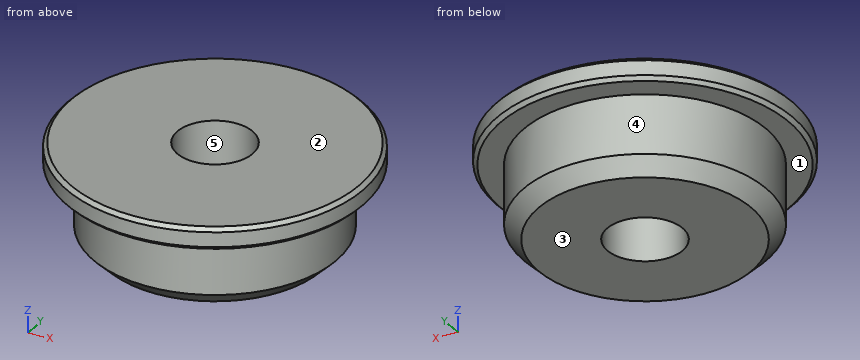
Autodesk Inventor part; units mm, degrees
ref_plane "YZ Plane" through (0, 0, 0) normal (1, 0, 0) x (0, 1, 0)
ref_plane "XZ Plane" through (0, 0, 0) normal (0, 1, 0) x (-1, 0, 0)
ref_plane "XY Plane" through (0, 0, 0) normal (0, 0, 1) x (1, 0, 0)
sketch "スケッチ1" plane through (0, 0, 0) normal (0, 0, 1) x (1, 0, 0)
  circle A0 centre (0, 0) radius 16.4
  dimension "d0" = 32.8
extrude "押し出し1" add sketch "スケッチ1" along normal blind 10
sketch "スケッチ2" plane through (0, 0, 10) normal (0, 0, 1) x (1, 0, 0)
  circle A0 centre (0, 0) radius 16.4
  circle A1 centre (0, 0) radius 20
  dimension "d3" = 40
extrude "押し出し2" add sketch "スケッチ2" along normal blind 3 contours A0 | A1
chamfer "面取り1" distance 2 angle 45 1 edges at (-16.4, 0, 0)
chamfer "面取り2" distance 0.5 angle 45 2 edges at (-20, 0, 13) (-20, 0, 10)
sketch "スケッチ3" plane through (0, 0, 13) normal (0, 0, 1) x (1, 0, 0)
  circle A0 centre (0, 0) radius 19.5
  circle A1 centre (0, 0) radius 5.1
  dimension "d12" = 10.2
extrude "押し出し3" cut sketch "スケッチ3" against normal through all contours A1
properties part number "Print_Parts_K" material "PC/ABS プラスチック"
Input: part model. Units: mm. Frame: model coordinates. Face numbers are marked on the shaded views. A direction names the side the tool comes from. Give positions to 0.01 mm unless a question says otherwise; leave off trailing zeros. Order: outer loops, then holes, each group sorted by start corner. A loop starts at its lowest first (then second) coordinate and runs counter-clockwise, first axis right, second up. Notation, with made-up numbers: (88, -27.5) - (132, -27.5) arc R23 ccw to (132, -5.5) - close; hole circle Ø3 at (1.25, -29.5). An arc over 180 degrees is marked (long way). One line per item, written item: value.
1. Line query: probe 1 along Y at (x, z) = (0, 5.5); probe 2 along Z at (x, y) = (9.5, 14); probe 3 along Y at (x, z) = (-3.5, 12). Output: solid intervals per line, ascending.
Determined:
probe 1: -16.4 to -5.1, 5.1 to 16.4
probe 2: 10 to 13
probe 3: -19.69 to -3.71, 3.71 to 19.69
2. Pin query (flat end, axial travel): pin 1 Ø2 at (y, z) = (-13.5, 10.5) entering from +X; pin 2 Ø3 at (y, z) = (11, 3.5) entering from +X; pin 3 Ø4 at (x, z) = (-5.5, 2.5) entering from -Y; pin 4 Ø16.5 at (x, y) = (0, 0) entering from +Z. Return the tip coordinate at first contact, or that it passes through.
Determined:
pin 1: x = 15.61
pin 2: x = 13.37
pin 3: y = -16.02
pin 4: z = 13
3. Reachability of the marked faces 1 and 2 from +Z, -Z, +X, -X, +Y, -Y: full face, straight path, thin tool, end or side. Return the list, or none.
Determined:
face 1: -Z
face 2: +Z, +X, -X, +Y, -Y
4. Cut plane B-B, the plane z = 8.5. Output: boundary loops of the cut face in (x, y).
Determined:
outline: circle Ø32.8 at (0, 0); hole circle Ø10.2 at (0, 0)
5. Draft query along Y for the marked faces 3, 4 and 5. Return one class per face: released by +Y, released by -Y, zero draft, split by the parting line, or undercut.
Determined:
face 3: zero draft
face 4: split by the parting line
face 5: undercut
6. Cut plane A-A, the plane x = 0. Output: boundary loops of the cut face in (y, z).
Determined:
outline: (-20, 10.5) - (-19.5, 10) - (-16.4, 10) - (-16.4, 2) - (-14.4, 0) - (-5.1, 0) - (-5.1, 13) - (-19.5, 13) - (-20, 12.5) - close; (5.1, 0) - (14.4, 0) - (16.4, 2) - (16.4, 10) - (19.5, 10) - (20, 10.5) - (20, 12.5) - (19.5, 13) - (5.1, 13) - close
